Part model, mm, in its own coordinate system. Face numbers are marked on the shaded views. Coordinates: 2 decimals unless noted, no trailing zeros. Use a Markdown table: item, result. Add a question column.
Q1. Wall check: L1, parallel to Z at x = 0, y = -1.8; L2, parallel to Z at x = 0, y = -6.1; L3, parallel to Z at x = 0, y = -0.4. Give the ranges that are in metal, low to high. Write a range as from..to.
Q2. Pin check, flat tips, straight feed: pin 1 Ø5 at (x, y) = (46, -1.5) entering from -Z; pin 2 Ø1.5 at (x, z) = (-5.5, -30) entering from -Y; pin 3 Ø2.5 at (x, y) = (33.5, -2.5) entering from +Z. Stop position of each tip, or through.
Q3. Mould opens along X. For the marked faces 1 and 2 say: released by +X, released by -X, zero draft, split by the parting line, or undercut.
from build123d import *

# Parameters (mm, degrees)
F0_R     = 62.5
F0_R_2   = 2.5
F1_DEPTH = 5
F2_R     = 1
F0_R_3   = 72.5
F3_DEPTH = 10
F4_R     = 2


with BuildPart() as f1:
    # F0 (on Front) → F1 (new body)
    with BuildSketch(Plane.XZ):
        Circle(F0_R)
        with BuildLine():
            ThreePointArc((-1.5, -10), (0, -8.5), (1.5, -10))
            Line((1.5, -10), (1.5, -55))
            ThreePointArc((1.5, -55), (0, -56.5), (-1.5, -55))
            Line((-1.5, -55), (-1.5, -10))
        make_face(mode=Mode.SUBTRACT)
        with BuildLine():
            ThreePointArc((-10, 1.5), (-8.5, 0), (-10, -1.5))
            Line((-10, -1.5), (-55, -1.5))
            ThreePointArc((-55, -1.5), (-56.5, 0), (-55, 1.5))
            Line((-55, 1.5), (-10, 1.5))
        make_face(mode=Mode.SUBTRACT)
        Circle(F0_R_2, mode=Mode.SUBTRACT)
        with BuildLine():
            Line((55, -1.5), (10, -1.5))
            ThreePointArc((10, -1.5), (8.5, 0), (10, 1.5))
            Line((10, 1.5), (55, 1.5))
            ThreePointArc((55, 1.5), (56.5, 0), (55, -1.5))
        make_face(mode=Mode.SUBTRACT)
        with BuildLine():
            Line((1.5, 55), (1.5, 10))
            ThreePointArc((1.5, 10), (0, 8.5), (-1.5, 10))
            Line((-1.5, 10), (-1.5, 55))
            ThreePointArc((-1.5, 55), (0, 56.5), (1.5, 55))
        make_face(mode=Mode.SUBTRACT)
    extrude(amount=F1_DEPTH)

    # F2
    f2_edges = [f1.edges().sort_by_distance(p)[0] for p in [
        (-62.5, -5, 0),
        (-62.5, 0, 0),
    ]]
    fillet(f2_edges, radius=F2_R)

    # F0 (on Front) → F3 (join)
    with BuildSketch(Plane.XZ):
        Circle(F0_R_3)
        Circle(F0_R, mode=Mode.SUBTRACT)
    extrude(amount=F3_DEPTH)

    # F4
    f4_edges = [f1.edges().sort_by_distance(p)[0] for p in [
        (-61.5, -5, 0),
        (-62.5, -10, 0),
        (-72.5, -10, 0),
        (-72.5, 0, 0),
    ]]
    fillet(f4_edges, radius=F4_R)


solid = f1.part
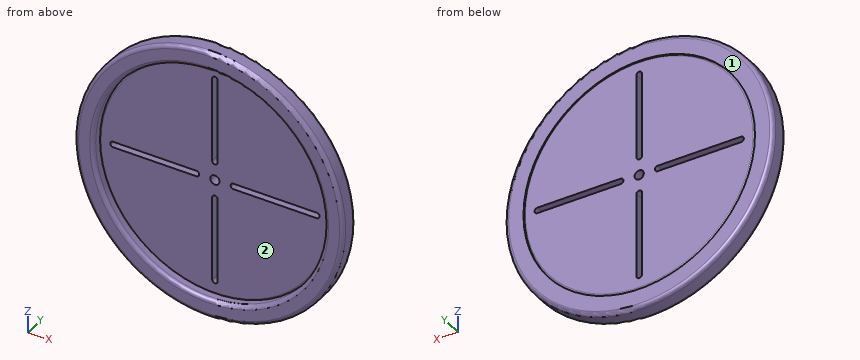
Recorded:
| question | item | result |
|---|---|---|
| 1 | L1 | -72.49..-56.5, -8.5..-2.5, 2.5..8.5, 56.5..72.49 |
| 1 | L2 | -72.5..-62.5, 62.5..72.5 |
| 1 | L3 | -71.7..-62.5, -62.3..-56.5, -8.5..-2.5, 2.5..8.5, 56.5..62.3, 62.5..71.7 |
| 2 | pin 1 | z = -57.97 |
| 2 | pin 2 | y = -5 |
| 2 | pin 3 | z = 64.93 |
| 3 | face 1 | zero draft |
| 3 | face 2 | undercut |
